Here's how the part is built. I have some questions about the finished solid (model axes, mm). Face numbers are marked on the shaded views. A direction names the side the tool comes from. Coordinates: 2 decimals unless noted, no trailing zeros. Order: outer loops, then holes, each group sorted by start corner. A loop starts at its lowest first (then second) coordinate and runs counter-clockwise, first axis right, second up. Notation, with made-up numbers: (71, -36) - (96, -36) arc R23 cw to (96, -14) - close; hole circle Ø2 at (-9, 1). An arc over 180 degrees is marked (long way). Answer as CSV lines item,"result". Start each with the question number.
Item 1: Imagine slicing it at C-C on z = -26.25. Count the separate pieces of the cut face and the enclosed holes in it, and give its area (3 significant figures).
Item 2: We'd pull the mould along Z, two halves only. Please class the marked faces 3, 4 and 5: pulls with the +Z half, pulls with the -Z half, needs draft (parallel to the pull), parting line crosses it, or undercut.
Item 3: On a 3-axis mill with a long thin cutter (end or side, diameter ignored), from which of +Z, -Z, +X, -X, +Y, -Y can I reach the whole of each face in a straight line? I mean the marked faces 1 and 2. Say none if no direction works.
Item 4: Imagine slicing it at A-A on y = -8.75. List the corners of the cut face in (x, z) for me, and give its area (3 significant figures).
Item 5: Imagine slicing it at B-B on y = -3.5. List the corners of the cut face in (x, z) for me.
Item 6: I'm going to push flat-ended pins straight in: pin 1 (10 mm diameter, centred on x = 26.25, z = 26.25, fed in from +Y); pin 2 (4.5 mm diameter, centred on x = 33.5, z = -1, fed in from -Y); pin 3 (3 mm diameter, centred on y = -4, z = 36, fed in from -X); pin 4 (5 mm diameter, centred on x = -26.25, z = -26.25, fed in from -Y). Where does each tip first touch, or does it pass through?
Item 7: I need wall thicknesses on line 1 (X direction, y = -10.5, z = 26.25); line 2 (Z direction, x = -26.25, y = -11.5); line 3 (Z direction, x = 0, y = -7). Which ranges of each line are inside material? Lowest first, please.
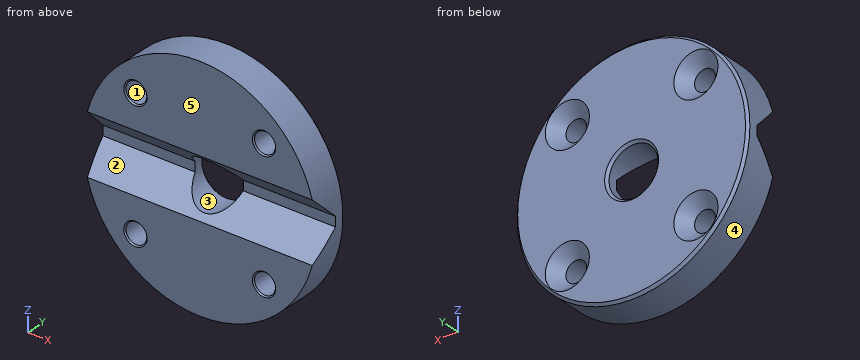
Autodesk Inventor part; units mm, degrees
ref_plane "YZ Plane" through (0, 0, 0) normal (1, 0, 0) x (0, 1, 0)
ref_plane "XZ Plane" through (0, 0, 0) normal (0, 1, 0) x (-1, 0, 0)
ref_plane "XY Plane" through (0, 0, 0) normal (0, 0, 1) x (1, 0, 0)
sketch "Sketch1" plane through (0, 0, 0) normal (0, 1, 0) x (-1, 0, 0)
  circle A0 centre (0, 0) radius 47.5
  circle A1 centre (0, 0) radius 10
  line L0 (-26.25, 26.25) -> (26.25, 26.25) construction
  line L1 (26.25, 26.25) -> (26.25, -26.25) construction
  line L2 (26.25, -26.25) -> (-26.25, -26.25) construction
  line L3 (-26.25, -26.25) -> (-26.25, 26.25) construction
  line L4 (-26.25, 26.25) -> (26.25, -26.25) construction
  line L5 (26.25, 26.25) -> (-26.25, -26.25) construction
  dimension "d0" = 95
  dimension "d1" = 20
  dimension "d33" = 52.5
extrude "Extrusion1" add sketch "Sketch1" against normal blind 15
hole "Hole1" at (-26.25, 0, -26.25) at (26.25, 0, -26.25) at (26.25, 0, 26.25) at (-26.25, 0, 26.25) direction (0, -1, 0) diameter 8.5 end through all countersink diameter 18 countersink angle 90
sketch "Sketch2" plane through (0, 0, 0) normal (1, 0, 0) x (0, 1, 0)
  line L0 (-15, 47.5) -> (-15, -47.5)
  line L1 (0, -47.5) -> (0, 47.5) construction
  line L2 (0, 47.5) -> (-15, 47.5) construction
  line L3 (0, -47.5) -> (-15, -47.5) construction
  line L4 (-46.8, 0) -> (7.8, 0) construction
  circle A0 centre (-24, 0) radius 15 construction
  line L5 (-15, 12.2132) -> (-4.7868, 2)
  line L6 (-4.7868, 2) -> (-4.7868, -2)
  line L7 (-4.7868, -2) -> (-15, -12.2132)
  point P0 (0, 0)
  point P1 (-4.7868, 0)
  dimension "d12" = 30
  dimension "d13" = 6
  dimension "d14" = 45
  dimension "d15" = 4
extrude "Extrusion2" cut sketch "Sketch2" along normal through all both and the other way through all
chamfer "Chamfer1" distance 1 angle 45 2 edges at (10, 0, 0) (47.5, 0, 0)
chamfer "Chamfer3" distance 0.5 angle 45 4 edges at (26.25, -15, -30.5) (-26.25, -15, -30.5) (26.25, -15, 22) (-26.25, -15, 22)
sketch "Sketch3" plane through (45.903, -15, 12.2132) normal (0, -0.7071, -0.7071) x (-1, 0, 0)
  ellipse E0 centre (45.903, 17.2721) end of major axis (45.903, 3.1299) minor radius 10 (36.1051, 14.4437) -> (55.701, 14.4437) ccw construction
  line L0 (-1.5549, 14.4437) -> (36.1051, 14.4437) construction
  ellipse E1 centre (45.903, 17.2721) end of major axis (45.903, 84.4472) minor radius 47.5 (-1.5549, 14.4437) -> (0, 0) ccw construction
  line L1 (91.806, 0) -> (0, 0) construction
  ellipse E2 centre (45.903, 17.2721) end of major axis (45.903, 84.4472) minor radius 47.5 (91.806, 0) -> (93.3609, 14.4437) ccw construction
  line L2 (55.701, 14.4437) -> (93.3609, 14.4437) construction
  line L3 (92.6036, 5) -> (-0.7976, 5)
  line L4 (93.1239, 10) -> (-1.3178, 10)
  line L5 (-1.5549, 14.4437) -> (93.3609, 14.4437)
  point P0 (45.903, 19.2426)
  dimension "d27" = 5
  dimension "d30" = 5
  dimension "d31" = 4.4436
sketch "Sketch4" plane through (-45.903, -15, -12.2132) normal (0, -0.7071, 0.7071) x (1, 0, 0)
  ellipse E0 centre (45.903, 17.2721) end of major axis (45.903, -49.9031) minor radius 47.5 (-1.5549, 14.4437) -> (0, 0) ccw construction
  ellipse E1 centre (45.903, 17.2721) end of major axis (45.903, -49.9031) minor radius 47.5 (91.806, 0) -> (93.3609, 14.4437) ccw construction
  line L0 (92.6036, 5) -> (-0.7976, 5)
  line L1 (91.806, 0) -> (0, 0) construction
  line L2 (93.3609, 14.4437) -> (-1.5549, 14.4437)
  line L3 (-1.3178, 10) -> (93.1239, 10)
  point P0 (45.903, 19.2426)
  dimension "d29" = 5
  dimension "d32" = 5
equation "\"d33\" = holeL"
equation "\"d30\" = d27"
equation "\"d29\" = d27"
equation "\"d32\" = d27"
properties part number "HM1_FIXT1-002"
Responses:
1,separate pieces,"3"
1,enclosed holes,"0"
1,area,"886 mm^2"
2,face 3,"undercut"
2,face 4,"parting line crosses it"
2,face 5,"needs draft"
3,face 1,"+Y, -Y"
3,face 2,"+X, -X, -Y"
4,outline,"(-47.12, -5.96) arc R47.5 ccw to (47.12, -5.96) - (8.03, -5.96) arc R10 cw to (-8.03, -5.96) - close; (-47.12, 5.96) - (-8.03, 5.96) arc R10 cw to (8.03, 5.96) - (47.12, 5.96) arc R47.5 ccw to start; hole circle Ø8.5 at (-26.25, -26.25); hole circle Ø8.5 at (-26.25, 26.25); hole circle Ø8.5 at (26.25, -26.25); hole circle Ø8.5 at (26.25, 26.25)"
4,area,"5,640 mm^2"
5,outline,"circle Ø95 at (0, 0); hole circle Ø11 at (-26.25, -26.25); hole circle Ø11 at (-26.25, 26.25); hole circle Ø20 at (0, 0); hole circle Ø11 at (26.25, -26.25); hole circle Ø11 at (26.25, 26.25)"
6,pin 1,"stops at y = -4"
6,pin 2,"stops at y = -6.04"
6,pin 3,"stops at x = -32.65"
6,pin 4,"passes through"
7,line 1,"x = -39.59 to -30.5, -22 to 22, 30.5 to 39.59"
7,line 2,"z = -39.59 to -30.5, -22 to -8.71, 8.71 to 22, 30.5 to 39.59"
7,line 3,"z = -47.5 to -10, 10 to 47.5"
